Part model, mm, in its own coordinate system. Face numbers are marked on the shaded views. A direction names the side the tool comes from. Round coordinates to 2 decimals unless told otherwise and drop trailing zeros. Loops run counter-clockwise (first coordinate to the right, second up) from the corner with the lowest first, then second, coordinate; pieces in that order, holes last.
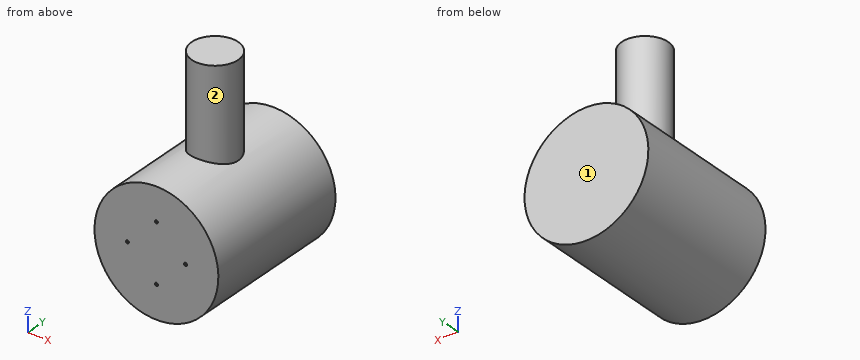
from build123d import *

# Parameters (mm, degrees)
SKETCH_1_R               = 80
EXTRUDE_1_DEPTH          = 200
SKETCH_2_R               = 30
EXTRUDE_2_DEPTH          = 195
SKETCH_3_R               = 2
CUT_EXTRUDE_1_DEPTH      = 2
PATTERN_CIRCULAR_1_COUNT = 4


with BuildPart() as part:
    # 草图1 → 凸台-拉伸1 (new body)
    with BuildSketch(Plane(origin=(0, 0, 0), x_dir=(1, 0, 0), z_dir=(0, 1, 0))):
        with Locations(Location((0, 0, 0), (0, 0, 270))):
            Circle(SKETCH_1_R)
    extrude(amount=EXTRUDE_1_DEPTH)

    # 草图2 → 凸台-拉伸2 (add)
    with BuildSketch(Plane.XY):
        with Locations(Location((0, 100, 0), (0, 0, 180))):
            Circle(SKETCH_2_R)
    extrude(amount=EXTRUDE_2_DEPTH)

    # 草图3 → 切除-拉伸1 (cut)
    with BuildSketch(Plane.XZ):
        with Locations(Location((0, 37.5, 0), (0, 0, 270))):
            Circle(SKETCH_3_R)
    cut_extrude_1 = extrude(amount=-CUT_EXTRUDE_1_DEPTH, mode=Mode.SUBTRACT)

    # 阵列(圆周)1: 切除-拉伸1 ×4 about axis
    pattern_circular_1_axis = Axis((0, 0, -0.023452158), (0, 1, 0))
    for i in range(1, PATTERN_CIRCULAR_1_COUNT):
        add(cut_extrude_1.rotate(pattern_circular_1_axis, i * 360 / PATTERN_CIRCULAR_1_COUNT), mode=Mode.SUBTRACT)


solid = part.part
1) Slice it at B-B, the plane y = 169.5. Give the cut face in (x, z).
Values:
outline: circle Ø160 at (0, 0)
2) Tool access for the marked faces 1 and 2: list every direction of +Z, -Z, +X, -X, +Y, -Y with a clear straight run to the whole face (end or side of a thin tool).
Values:
face 1: +Z, -Z, +X, -X, +Y
face 2: +Z
3) Drop flat-ended pins along their axis: pin 1 Ø6 at (x, z) = (7, 88) entering from -Y; pin 2 Ø2 at (y, z) = (96.5, 56.5) entering from -X; pin 3 Ø10 at (y, z) = (23, 21) entering from -X; pin 4 Ø5 at (x, z) = (0, -37.55) entering from -Y. Give the stop position or say it passes through.
Values:
pin 1: stops at y = 70.27
pin 2: stops at x = -57.62
pin 3: stops at x = -78.38
pin 4: stops at y = 0
4) Slice it at A-A, the plane x = 22. Give the cut face in (y, z).
Values:
outline: (0, -76.92) - (200, -76.92) - (200, 76.92) - (120.4, 76.92) - (120.4, 195) - (79.6, 195) - (79.6, 76.92) - (0, 76.92) - close
5) Slice it at D-D, the plane y = 100. Give the cut face in (x, z), then the cut area to 3 significant figures.
Values:
outline: (-30, 74.16) arc R80 ccw (long way) to (30, 74.16) - (30, 195) - (-30, 195) - close
area: 27,100 mm2
6) Wall check: line 1 along X through (y, z) = (161, -29.5); line 2 along Z through (x, y) = (9.5, 115); line 3 along Z through (x, y) = (30.5, 9.5). Give the ranges that are in metal, low to high.
Values:
line 1: x = -74.36 to 74.36
line 2: z = -79.43 to 195
line 3: z = -73.96 to 73.96
7) Slice it at C-C, the plane z = -44. Give the cut face in (x, y), then the cut area to 3 significant figures.
Values:
outline: (-66.81, 0) - (66.81, 0) - (66.81, 200) - (-66.81, 200) - close
area: 26,700 mm2
